Part model, mm, in its own coordinate system. Give positions to 0.01 mm unless a question says otherwise; leave off trailing zeros. Write item = value, one per line. Start each with the question number.
from build123d import *

# Parameters (mm, degrees)
SKETCH1_W               = 162
SKETCH1_H               = 162
BOSS_EXTRUDE1_DEPTH     = 5.5
SKETCH2_R               = 2.65
CUT_EXTRUDE1_DEPTH      = 10
MIRROR2_COPY_1_SKETCH_R = 2.65
MIRROR2_COPY_1_DEPTH    = 10
FILLET1_R               = 10


with BuildPart() as part:
    # Sketch1 → Boss-Extrude1 (new, symmetric)
    with BuildSketch(Plane(origin=(0, 0, 0), x_dir=(1, 0, 0), z_dir=(0, 1, 0))):
        Rectangle(SKETCH1_W, SKETCH1_H)
    extrude(amount=BOSS_EXTRUDE1_DEPTH, both=True)

    # Sketch2 → Cut-Extrude1 (cut)
    with BuildSketch(Plane(origin=(0, 5.5, 0), x_dir=(1, 0, 0), z_dir=(0, 1, 0))):
        with Locations(Location((9, -9, 0), (0, 0, 270))):
            Circle(SKETCH2_R)
        with Locations(Location((27, -9, 0), (0, 0, 270))):
            Circle(SKETCH2_R)
        with Locations(Location((45, -9, 0), (0, 0, 270))):
            Circle(SKETCH2_R)
        with Locations(Location((63, -9, 0), (0, 0, 270))):
            Circle(SKETCH2_R)
        with Locations(Location((9, -27, 0), (0, 0, 270))):
            Circle(SKETCH2_R)
        with Locations(Location((27, -27, 0), (0, 0, 270))):
            Circle(SKETCH2_R)
        with Locations(Location((45, -27, 0), (0, 0, 270))):
            Circle(SKETCH2_R)
        with Locations(Location((63, -27, 0), (0, 0, 270))):
            Circle(SKETCH2_R)
        with Locations(Location((9, -45, 0), (0, 0, 270))):
            Circle(SKETCH2_R)
        with Locations(Location((27, -45, 0), (0, 0, 270))):
            Circle(SKETCH2_R)
        with Locations(Location((45, -45, 0), (0, 0, 270))):
            Circle(SKETCH2_R)
        with Locations(Location((63, -45, 0), (0, 0, 270))):
            Circle(SKETCH2_R)
        with Locations(Location((9, -63, 0), (0, 0, 270))):
            Circle(SKETCH2_R)
        with Locations(Location((27, -63, 0), (0, 0, 270))):
            Circle(SKETCH2_R)
        with Locations(Location((45, -63, 0), (0, 0, 270))):
            Circle(SKETCH2_R)
        with Locations(Location((63, -63, 0), (0, 0, 270))):
            Circle(SKETCH2_R)
    cut_extrude1 = extrude(amount=-CUT_EXTRUDE1_DEPTH, mode=Mode.SUBTRACT)

    # Mirror1: Cut-Extrude1 across plane
    add(cut_extrude1.mirror(Plane.XY), mode=Mode.SUBTRACT)

    # Mirror2: Cut-Extrude1 across plane
    add(cut_extrude1.mirror(Plane(origin=(0, 0, 0), x_dir=(0, 0, 1), z_dir=(1, 0, 0))), mode=Mode.SUBTRACT)

    # Mirror2 copy 1 sketch → Mirror2 copy 1 (cut)
    with BuildSketch(Plane(origin=(0, 5.5, 0), x_dir=(-1, 0, 0), z_dir=(0, 1, 0))):
        with Locations(Location((9, -9, 0), (0, 0, 270))):
            Circle(MIRROR2_COPY_1_SKETCH_R)
        with Locations(Location((27, -9, 0), (0, 0, 270))):
            Circle(MIRROR2_COPY_1_SKETCH_R)
        with Locations(Location((45, -9, 0), (0, 0, 270))):
            Circle(MIRROR2_COPY_1_SKETCH_R)
        with Locations(Location((63, -9, 0), (0, 0, 270))):
            Circle(MIRROR2_COPY_1_SKETCH_R)
        with Locations(Location((9, -27, 0), (0, 0, 270))):
            Circle(MIRROR2_COPY_1_SKETCH_R)
        with Locations(Location((27, -27, 0), (0, 0, 270))):
            Circle(MIRROR2_COPY_1_SKETCH_R)
        with Locations(Location((45, -27, 0), (0, 0, 270))):
            Circle(MIRROR2_COPY_1_SKETCH_R)
        with Locations(Location((63, -27, 0), (0, 0, 270))):
            Circle(MIRROR2_COPY_1_SKETCH_R)
        with Locations(Location((9, -45, 0), (0, 0, 270))):
            Circle(MIRROR2_COPY_1_SKETCH_R)
        with Locations(Location((27, -45, 0), (0, 0, 270))):
            Circle(MIRROR2_COPY_1_SKETCH_R)
        with Locations(Location((45, -45, 0), (0, 0, 270))):
            Circle(MIRROR2_COPY_1_SKETCH_R)
        with Locations(Location((63, -45, 0), (0, 0, 270))):
            Circle(MIRROR2_COPY_1_SKETCH_R)
        with Locations(Location((9, -63, 0), (0, 0, 270))):
            Circle(MIRROR2_COPY_1_SKETCH_R)
        with Locations(Location((27, -63, 0), (0, 0, 270))):
            Circle(MIRROR2_COPY_1_SKETCH_R)
        with Locations(Location((45, -63, 0), (0, 0, 270))):
            Circle(MIRROR2_COPY_1_SKETCH_R)
        with Locations(Location((63, -63, 0), (0, 0, 270))):
            Circle(MIRROR2_COPY_1_SKETCH_R)
    extrude(amount=-MIRROR2_COPY_1_DEPTH, mode=Mode.SUBTRACT)

    # Fillet1
    fillet1_edges = [part.edges().sort_by_distance(p)[0] for p in [
        (81, 0, 81),
        (-81, 0, 81),
        (-81, 0, -81),
        (81, 0, -81),
    ]]
    fillet(fillet1_edges, radius=FILLET1_R)


solid = part.part
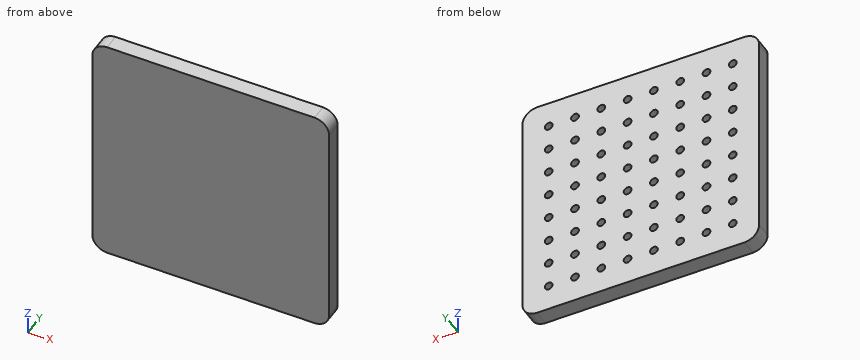
Q1. Drop a flat-ended pin along its axis: P1, Ø1.6, axis at x = -64, z = -25.5, coming from the +Y side. Give the stop position or say it passes through.
Q2. Slice it at A-A (y = 1). Give the number of separate pieces and of enclosed holes in the cut face, and give its area (3 significant figures).
Q3. Probe line 1 along Y through (x, z) = (43, -26.5); line 2 along X through (y, z) = (2, -74). List the from-to ranges inside material, lowest first.
Working result:
q1.P1 = -4.5
q2.separate_pieces = 1
q2.enclosed_holes = 64
q2.area = 24,700 mm2
q3.line_1 = -5.5 to -4.5
q3.line_2 = -80.54 to 80.54
